Source: three-view drawing plus pictorial views. Frame: mm from the lowest corner of the part. A direction names the side the tool comes from. Give positions to 0.01 mm unless a question says otherwise; leave off trailing zeros. Order: outer loops, then holes, each group sorted by start corner. A loop starts at its lowest first (then second) coordinate and runs counter-clockwise, first axis right, second up. Notation, with made-up numbers: (-24, 54) - (9, 54) arc R10 cw to (9, 65) - close; hole circle Ø10 at (-21.75, 13). An arc over 180 degrees is marked (long way). Answer in a Markdown table with one row per item. Add a question column.
1. Access query for the marked faces 1 and 2. Directions: +Z, -Z, +X, -X, +Y, -Y. A direction counts if a zero-diameter tool reaches every point of the face in a straight line with its end or side. Return the directions, or none.
2. Section query A-A on x = 45. Return loops of the section in (y, z).
3. Section query B-B on y = 19. Return loops of the section in (x, z).
4. Contact query for flat-ended pins moving along their axis: pin 1 (3.5 mm diameter, centred on x = 30, y = 19, fed in from -Z); pin 2 (3 mm diameter, centred on x = 44.5, z = 4, fed in from -Y); pin 3 (12 mm diameter, centred on x = 32.5, y = 12.5, fed in from -Z). Output: stop coordinate, or through.
5. Ray query, line 1 (X direction, y = 23.95, z = 7.5); line 2 (Y direction, x = 30, z = 24.3); line 3 (Z direction, x = 45, y = 23.95). Return the intervals inside material, ascending. Write a range as [from, to].
6. Section query C-C on z = 7.5. Return loops of the section in (x, y).
7. Section query D-D on x = 5. Return loops of the section in (y, z), and give its area (3 significant figures).
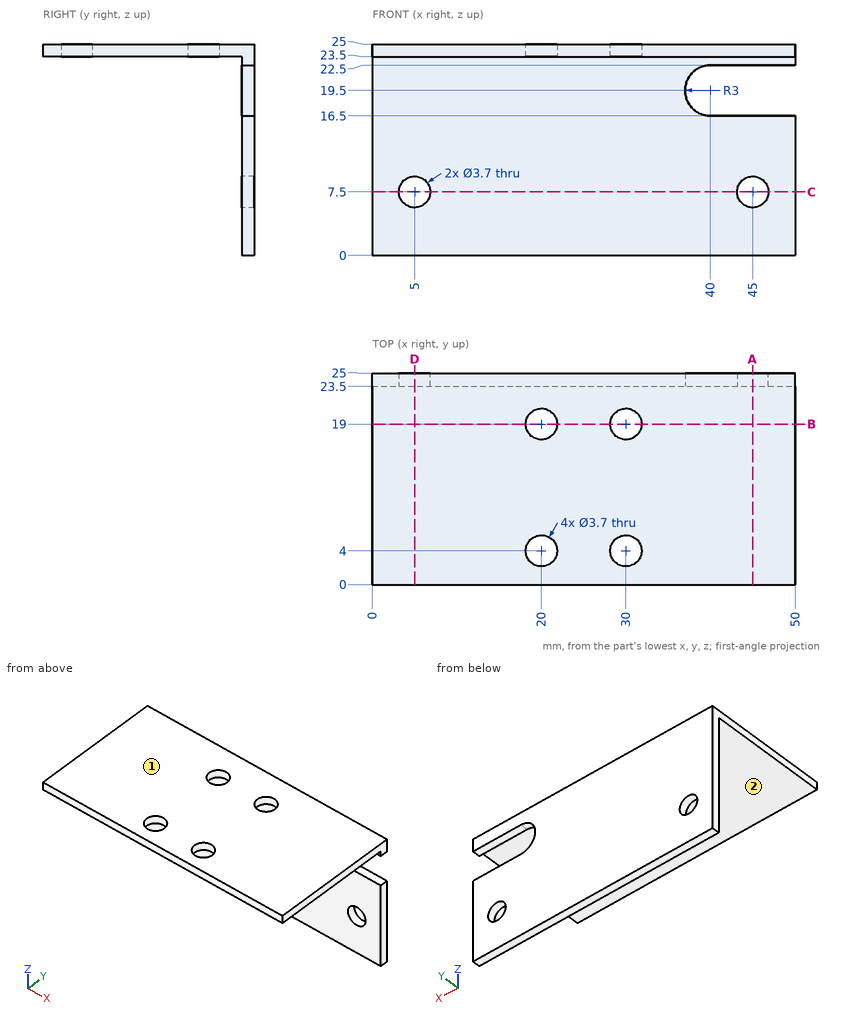
Answer:
| question | item | result |
|---|---|---|
| 1 | face 1 | +Z, +X, -X, +Y, -Y |
| 1 | face 2 | -Z, +X, -X, -Y |
| 2 | outline | (0, 23.5) - (23.5, 23.5) - (23.5, 22.5) - (25, 22.5) - (25, 25) - (0, 25) - close; (23.5, 0) - (25, 0) - (25, 5.65) - (23.5, 5.65) - close; (23.5, 9.35) - (25, 9.35) - (25, 16.5) - (23.5, 16.5) - close |
| 3 | outline | (0, 23.5) - (18.15, 23.5) - (18.15, 25) - (0, 25) - close; (21.85, 23.5) - (28.15, 23.5) - (28.15, 25) - (21.85, 25) - close; (31.85, 23.5) - (50, 23.5) - (50, 25) - (31.85, 25) - close |
| 4 | pin 1 | passes through |
| 4 | pin 2 | stops at y = 23.5 |
| 4 | pin 3 | stops at z = 23.5 |
| 5 | line 1 | x = [0, 3.15], [6.85, 43.15], [46.85, 50] |
| 5 | line 2 | y = [0, 2.15], [5.85, 17.15], [20.85, 25] |
| 5 | line 3 | z = [0, 5.65], [9.35, 16.5], [22.5, 25] |
| 6 | outline | (0, 23.5) - (3.15, 23.5) - (3.15, 25) - (0, 25) - close; (6.85, 23.5) - (43.15, 23.5) - (43.15, 25) - (6.85, 25) - close; (46.85, 23.5) - (50, 23.5) - (50, 25) - (46.85, 25) - close |
| 7 | outline | (0, 23.5) - (23.5, 23.5) - (23.5, 9.35) - (25, 9.35) - (25, 25) - (0, 25) - close; (23.5, 0) - (25, 0) - (25, 5.65) - (23.5, 5.65) - close |
| 7 | area | 67.2 mm² |
